from build123d import *

# Parameters (mm, degrees)
F1_DEPTH      = 40
F3_DEPTH      = 25.2082594216
F3_DEPTH_BACK = 25


with BuildPart() as f1:
    # F0 (on Top) → F1 (new body)
    with BuildSketch(Plane.XY):
        Polygon((-5, 0), (0, 0), (25.4034118443, 44), (9.7927405784, 44), (9.7927405784, 40), (0, 40), (-25.2072594216, 40), (-5, 5), align=None)
    extrude(amount=F1_DEPTH)

    # F2 (on Right) → F3 (cut, two sides)
    with BuildSketch(Plane.YZ) as f3_sk:
        Polygon((35, 40), (0, 40), (0, 19.7927405784), align=None)
    extrude(amount=-F3_DEPTH, mode=Mode.SUBTRACT)
    extrude(f3_sk.sketch, amount=F3_DEPTH_BACK, mode=Mode.SUBTRACT)


solid = f1.part
CAD build for the part. Positions are in the model's coordinates, mm. A direction names the side the tool comes from. Coordinates: 2 decimals unless noted, no trailing zeros. Write each loop counter-clockwise with the first axis right and the second up, starting at its lowest first coordinate (ties: lowest second). Pieces come first, ordered by that corner, then holes. Notation, with made-up numbers: M 35.25,-4 L 68.25,-4 A28 cw 68.25,19 Z; hole C -26,64.25 d10. An arc over 180 degrees is marked long. Answer as a JSON object with one key per item and string values. Group by question number.
1) Wall check: line 1 (Y direction, x = -4, z = 6); line 2 (Y direction, x = 14, z = 29.5); line 3 (X direction, y = 36, z = 26.5). Give the ranges that are in metal, low to high. Write a range as from..to.
2) Tool access for faces 1 (the face through (-7, 40, 20)), 2 (the face through (-5, 3, 11)), 3 (the face through (0, 27, 0)): list every direction of +Z, -Z, +X, -X, +Y, -Y with a clear straight run to the whole face (end or side of a thin tool).
3) Pin check, flat tips, straight feed: pin 1 Ø5 at (y, z) = (22, 8.5) entering from -X; pin 2 Ø1.5 at (y, z) = (3.5, 8.5) entering from -X; pin 3 Ø12 at (x, y) = (8, 19) entering from +Z; pin 4 Ø6 at (x, y) = (15, 16.5) entering from -Z. Stop position of each tip, or through.
4) Saw through at C-C (y = 32). Write the cut outline in (x, z), plus the area to 3 significant figures.
5) Saw through at D-D (x = -15). Write the cut outline in (y, z).
6) Saw through at A-A (z = 27). Write the cut outline in (x, y), plus the area to 3 significant figures.
7) Saw through at B-B (x = 9). Write the cut outline in (y, z), plus the area to 3 significant figures.
Values follow:
{
 "1": {"line 1": "y = 0..40", "line 2": "y = 24.25..44", "line 3": "x = -22.9..20.78"},
 "2": {"face 1": "+Z, -Z, -X, +Y", "face 2": "+Z, -Z, -X, -Y", "face 3": "-Z, +X, -X, +Y, -Y"},
 "3": {"pin 1": "stops at x = -16.26", "pin 2": "stops at x = -5", "pin 3": "stops at z = 34.23", "pin 4": "passes through"},
 "4": {"outline": "M -20.59,0 L 18.48,0 L 18.48,38.27 L -20.59,38.27 Z", "area": "1,490 mm2"},
 "5": {"outline": "M 22.32,0 L 40,0 L 40,40 L 35,40 L 22.32,32.68 Z"},
 "6": {"outline": "M -25.21,40 L -9.32,12.48 L 7.21,12.48 L 25.4,44 L 9.79,44 L 9.79,40 Z", "area": "950 mm2"},
 "7": {"outline": "M 15.59,0 L 40,0 L 40,40 L 35,40 L 15.59,28.79 Z", "area": "868 mm2"}
}
